CAD build for the part. Positions are in the model's coordinates, mm. Give positions to 0.01 mm unless a question says otherwise; leave off trailing zeros. Write each loop counter-clockwise with the first axis right and the second up, starting at its lowest first coordinate (ties: lowest second). Pieces come first, ordered by that corner, then holes. Notation, with made-up numbers: (57, 35.5) -> (107, 35.5) arc R21 cw to (107, 44.5) -> close; hole circle Ø3 at (76, 20). An arc over 180 degrees is marked (long way). Use one line per item in the form item = value. Start each with the question number.
from build123d import *

# Parameters (mm, degrees)
F0_W     = 80
F0_H     = 95
F0_R     = 3
F1_DEPTH = 6


with BuildPart() as f1:
    # F0 (on Top) → F1 (new body)
    with BuildSketch(Plane.XY):
        Rectangle(F0_W, F0_H)
        with Locations((-23.6, -32.417263)):
            Circle(F0_R, mode=Mode.SUBTRACT)
        with Locations((23.6, -32.417263)):
            Circle(F0_R, mode=Mode.SUBTRACT)
        with Locations((-23.6, 14.782737)):
            Circle(F0_R, mode=Mode.SUBTRACT)
        with BuildLine():
            ThreePointArc((-20.5, 36.533368), (-18, 39.033368), (-15.5, 36.533368))
            Line((-15.5, 36.533368), (-15.5, 26.533368))
            ThreePointArc((-15.5, 26.533368), (-18, 24.033368), (-20.5, 26.533368))
            Line((-20.5, 26.533368), (-20.5, 36.533368))
        make_face(mode=Mode.SUBTRACT)
        with Locations((23.6, 14.782737)):
            Circle(F0_R, mode=Mode.SUBTRACT)
        with BuildLine():
            ThreePointArc((20.5, 26.533368), (18, 24.033368), (15.5, 26.533368))
            Line((15.5, 26.533368), (15.5, 36.533368))
            ThreePointArc((15.5, 36.533368), (18, 39.033368), (20.5, 36.533368))
            Line((20.5, 36.533368), (20.5, 26.533368))
        make_face(mode=Mode.SUBTRACT)
    extrude(amount=F1_DEPTH)


solid = f1.part
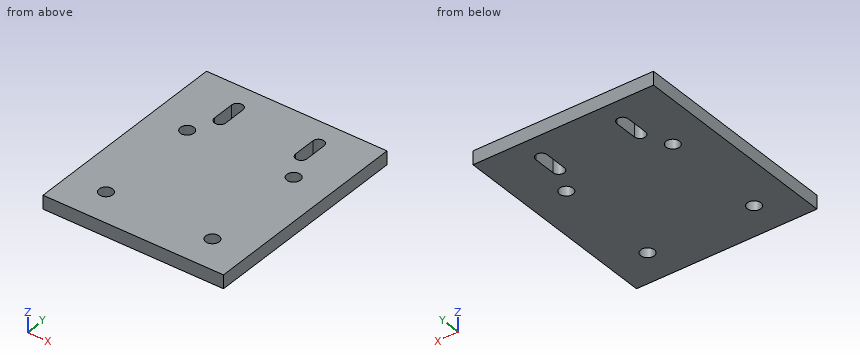
1) Cut at B-B (x = -23.6). Give the cut face in (y, z).
2) Wall check: line 1 along X through (y, z) = (35.5, 2.8); line 2 along Y through (x, z) = (23.6, 2.7); line 3 along X through (y, z) = (16.5, 2.4). Give the ranges that are in metal, low to high. Write a range as from..to.
3) Cut at C-C (z = 4.55). Give the cut face in (x, y), and give its area (3 significant figures).
4) Pin check, flat tips, straight feed: pin 1 (8 mm diameter, centred on x = -23.6, y = 14.78, fed in from -Z); pin 2 (5 mm diameter, centred on x = -23.6, y = -32.42, fed in from -Z). Stop position of each tip, or through.
5) Cut at A-A (x = 18). Give the cut face in (y, z).
Final values:
q1.outline = (-47.5, 0) -> (-35.42, 0) -> (-35.42, 6) -> (-47.5, 6) -> close; (-29.42, 0) -> (11.78, 0) -> (11.78, 6) -> (-29.42, 6) -> close; (17.78, 0) -> (47.5, 0) -> (47.5, 6) -> (17.78, 6) -> close
q2.line_1 = -40..-20.5, -15.5..15.5, 20.5..40
q2.line_2 = -47.5..-35.42, -29.42..11.78, 17.78..47.5
q2.line_3 = -40..-26.06, -21.14..21.14, 26.06..40
q3.outline = (-40, -47.5) -> (40, -47.5) -> (40, 47.5) -> (-40, 47.5) -> close; hole circle Ø6 at (-23.6, -32.42); hole circle Ø6 at (-23.6, 14.78); hole (-20.5, 26.53) arc R2.5 ccw to (-15.5, 26.53) -> (-15.5, 36.53) arc R2.5 ccw to (-20.5, 36.53) -> close; hole (15.5, 26.53) arc R2.5 ccw to (20.5, 26.53) -> (20.5, 36.53) arc R2.5 ccw to (15.5, 36.53) -> close; hole circle Ø6 at (23.6, -32.42); hole circle Ø6 at (23.6, 14.78)
q3.area = 7,350 mm^2
q4.pin_1 = 0
q4.pin_2 = through
q5.outline = (-47.5, 0) -> (24.03, 0) -> (24.03, 6) -> (-47.5, 6) -> close; (39.03, 0) -> (47.5, 0) -> (47.5, 6) -> (39.03, 6) -> close
